Check sheet for the modelled part. Datum: model origin and axes. Units: mm. A direction names the side the tool comes from. Give positions to 0.01 mm unless a question says otherwise; leave off trailing zeros. Order: outer loops, then holes, each group sorted by start corner. A loop starts at its lowest first (then second) coordinate and runs counter-clockwise, first axis right, second up.
```python
from build123d import *

# Parameters (mm, degrees)
CHANFREIN1_SIZE = 0.25


with BuildPart() as part:
    # Esquisse1 → Révolution1 (revolve)
    with BuildSketch(Plane(origin=(0, 0, 0), x_dir=(1, 0, 0), z_dir=(0, 1, 0)), mode=Mode.PRIVATE) as r_volution1_sk:
        Polygon((8, 5), (1, 5), (1, 6), (0, 6), (0, 4), (8, 4), align=None)
    revolve(r_volution1_sk.sketch.rotate(Axis((-2.315789474, 0, 0), (1, 0, 0)), 180), axis=Axis((-2.315789474, 0, 0), (1, 0, 0)))

    # Chanfrein1
    chanfrein1_edges = [part.edges().sort_by_distance(p)[0] for p in [
        (8, 0, -4),
        (0, 0, -4),
        (0, 0, -6),
        (1, 0, -6),
        (8, 0, -5),
    ]]
    chamfer(chanfrein1_edges, length=CHANFREIN1_SIZE)


solid = part.part
```
Q1. Draft check along Z on faces 1 (the cylindrical face through (0.496, -1.802, 5.723)), 2 (the flat face through (0, 4, -2)), 3 (the cylindrical face through (4.052, 3.905, -0.867)). Enter one of: pulls with the +Z half, pulls with the -Z half, needs draft (parallel to the pull), parting line crosses it, or undercut.
Q2. Sectioned sample at C-C, the plane x = 7.5. Record the cut outline in (y, z), plus the area to 3 significant figures.
Q3. Tool access check on faces 4 (the flat face through (8, 2, 4)), 5 (the flat face through (1, -5, 2)). Record the directions out of +Z, -Z, +X, -X, +Y, -Y that give a thin tool (end or side, any length) a straight path to the whole face; none if there is none.
Q4. Go/stop test with flat-tipped pins: P1, Ø4, axis at x = 4, y = -3.5, coming from the -Z side; P2, Ø3, axis at x = 4.5, z = -2.5, coming from the -Y side; P3, Ø1.5, axis at x = 2, y = -4, coming from the +Z side. Record where each tip stops, or that it passes through.
Q5. Sectioned sample at A-A, the plane y = 0. Record the cut outline in (x, z), plus the area to 3 significant figures.
Q6. Material ranges on line 1 (Y direction, x = 3.25, z = 0); line 2 (Y direction, x = 3.25, z = 3); line 3 (X direction, y = -1.25, z = 5.5), recorded low to high.
Filled in:
1. face 1: parting line crosses it
1. face 2: needs draft
1. face 3: undercut
2. outline: circle Ø10 at (0, 0); hole circle Ø8 at (0, 0)
2. area: 28.3 mm2
3. face 4: +Z, -Z, +X, +Y, -Y
3. face 5: +X
4. P1: stops at z = -4.77
4. P2: stops at y = -4.9
4. P3: stops at z = 3.8
5. outline: (0, -5.75) - (0.25, -6) - (0.75, -6) - (1, -5.75) - (1, -5) - (7.75, -5) - (8, -4.75) - (8, -4.25) - (7.75, -4) - (0.25, -4) - (0, -4.25) - close; (0, 4.25) - (0.25, 4) - (7.75, 4) - (8, 4.25) - (8, 4.75) - (7.75, 5) - (1, 5) - (1, 5.75) - (0.75, 6) - (0.25, 6) - (0, 5.75) - close
5. area: 17.7 mm2
6. line 1: y = -5 to -4, 4 to 5
6. line 2: y = -4 to -2.65, 2.65 to 4
6. line 3: x = 0 to 1
